from build123d import *

# Parameters (mm, degrees)
SKETCH1_R           = 7.9248
BOSS_EXTRUDE1_DEPTH = 38.1
CHAMFER1_SIZE       = 1.524
CHAMFER2_SIZE       = 1.524


with BuildPart() as part:
    # Sketch1 → Boss-Extrude1 (new body, symmetric)
    with BuildSketch(Plane(origin=(0, 0, 0), x_dir=(0, 0, -1), z_dir=(1, 0, 0))):
        Circle(SKETCH1_R)
    extrude(amount=BOSS_EXTRUDE1_DEPTH, both=True)

    # Chamfer1
    chamfer1_edges = [part.edges().sort_by_distance(p)[0] for p in [
        (38.1, 0, 7.9248),
    ]]
    chamfer(chamfer1_edges, length=CHAMFER1_SIZE)

    # Chamfer2
    chamfer2_edges = [part.edges().sort_by_distance(p)[0] for p in [
        (-38.1, 0, 7.9248),
    ]]
    chamfer(chamfer2_edges, length=CHAMFER2_SIZE)


solid = part.part
Design review of the part built by this model. Coordinates are the model's own, in mm. Round coordinates to 2 decimals unless told otherwise and drop trailing zeros. Write each loop counter-clockwise with the first axis right and the second up, starting at its lowest first coordinate (ties: lowest second). Pieces come first, ordered by that corner, then holes. Notation, with made-up numbers: (58, -4.5) -> (107, -4.5) arc R23 ccw to (107, 31.5) -> close; hole circle Ø5 at (63, 80.25). An arc over 180 degrees is marked (long way). One line per item, written item: value. Start each with the question number.
Q1. To check wall thickness, follow probe 1 along Z at (x, y) = (-21.5, -0.5); probe 2 along Y at (x, z) = (-5, -3.25); probe 3 along Y at (x, z) = (10, -2.25). State the ranges of each line that lie inside material, in increasing order.
Q2. Add section A-A (x = -32). Give the boundary of the cut face in (y, z), then the cut area to 3 significant figures.
Q3. Insertion check: P1, Ø3, axis at x = 6.5, y = -5.5, coming from the +Z side; P2, Ø4, axis at x = -19.5, y = 4.5, coming from the -Z side; P3, Ø1, axis at x = -30, y = -4, coming from the +Z side. Each pin has a flat end and moves straight along its axis. Give the tip position at first contact, or say it passes through.
Response:
1. probe 1: z = -7.91 to 7.91
1. probe 2: y = -7.23 to 7.23
1. probe 3: y = -7.6 to 7.6
2. outline: circle Ø15.85 at (0, 0)
2. area: 197 mm^2
3. P1: stops at z = 6.84
3. P2: stops at z = -7.52
3. P3: stops at z = 7.11
